The model under review builds one solid part; all positions refer to its coordinate system, in mm. A direction names the side the tool comes from. Give positions to 0.01 mm unless a question says otherwise; leave off trailing zeros. Order: outer loops, then holes, each group sorted by start corner. A loop starts at its lowest first (then second) coordinate and runs counter-clockwise, first axis right, second up. Notation, with made-up numbers: (21.5, 49.5) - (61.5, 49.5) arc R25 cw to (61.5, 61.5) - close; hole circle Ø8 at (16.25, 53.5). An arc over 180 degrees is marked (long way). Use CSV: the item, a comma, the result in double quotes. Start each with the question number.
1. For pin 1 (1 mm diameter, centred on x = -7, y = 484, fed in from +Z); pin 2 (5 mm diameter, centred on y = 8.5, z = -7.5, fed in from +X); pin 3 (5 mm diameter, centred on x = 5.5, y = 655, fed in from -Z), all flat-tipped, find the tip position at first contact; note any pin that passes through.
2. Take a section at B-B, the plane z = -6. State the section outline as (x, y) points (1 decimal), then the cut area to 3 significant figures.
3. To check wall thickness, follow line 1 (X direction, y = 816.5, z = -1.75); line 2 (Y direction, x = -0.75, z = -6.5); line 3 (Z direction, x = 0.5, y = 560). State the ranges of each line that lie inside material, in increasing order. Write a range as [from, to].
4. Machinability: for faces 4 (the flat face through (-4.762, 13, -3)), 5 (the flat face through (0, 0, 6)), which of the approach directions +Z, -Z, +X, -X, +Y, -Y give a long, thin tool a straight path to every point of the face, cutting with its end or side? Answer none if there is none.
5. Take a section at A-A, the plane x = 0. State the section outline as (y, z) points, then the cut area to 3 significant figures.
6. Draft analysis for pull direction X (two halves, no side actions). For faces 1 (the cylindrical face through (-2.75, 450.8, -12.4)), 2 (the flat face through (0, 914.4, 0)), 3 (the flat face through (4.762, 13, -4)), state which applies: released by +X, released by -X, zero draft, split by the parting line, or undercut.
7. Take a section at C-C, the plane y = 645.5. State the section outline as (x, z) points, then the cut area to 3 significant figures.
```python
from build123d import *

# Parameters (mm, degrees)
F0_R     = 12.7
F1_DEPTH = 914.4
F3_DEPTH = 25.4
F6_DEPTH = 17.4625


with BuildPart() as f1:
    # F0 (on Front) → F1 (new body)
    with BuildSketch(Plane.XZ):
        Circle(F0_R)
    extrude(amount=-F1_DEPTH)

    # F2 (on face) → F3 (cut)
    with BuildSketch(Plane.XZ):
        with BuildLine():
            Line((4.7625, 4.7625), (-4.7625, 4.7625))
            Line((-4.7625, 4.7625), (-4.7625, -11.773215))
            ThreePointArc((-4.7625, -11.773215), (0, -12.7), (4.7625, -11.773215))
            Line((4.7625, -11.773215), (4.7625, 4.7625))
        make_face()
    extrude(amount=-F3_DEPTH, mode=Mode.SUBTRACT)

    # F5 (on offset) → F6 (cut, through all)
    with BuildSketch(Plane.XY.offset(-12.7)):
        with BuildLine():
            ThreePointArc((4.7625, 25.4), (0, 30.1625), (-4.7625, 25.4))
            Line((-4.7625, 25.4), (4.7625, 25.4))
        make_face()
    extrude(amount=F6_DEPTH, mode=Mode.SUBTRACT)


solid = f1.part
```
Determined:
1,pin 1,"stops at z = 10.91"
1,pin 2,"stops at x = 11.67"
1,pin 3,"stops at z = -12.34"
2,outline,"(-11.2, 0) - (-4.8, 0) - (-4.8, 25.4) arc R4.8 cw to (4.8, 25.4) - (4.8, 0) - (11.2, 0) - (11.2, 914.4) - (-11.2, 914.4) - close"
2,area,"20,200 mm²"
3,line 1,"x = [-12.58, 12.58]"
3,line 2,"y = [30.1, 914.4]"
3,line 3,"z = [-12.69, 12.69]"
4,face 4,"-Z, -Y"
4,face 5,"+Z, -Z, +X, -X, -Y"
5,outline,"(0, 4.76) - (30.16, 4.76) - (30.16, -12.7) - (914.4, -12.7) - (914.4, 12.7) - (0, 12.7) - close"
5,area,"22,700 mm²"
6,face 1,"split by the parting line"
6,face 2,"zero draft"
6,face 3,"undercut"
7,outline,"circle Ø25.4 at (0, 0)"
7,area,"507 mm²"
